Can you work these out from the model? Positions are in its coordinate system, mm. Face numbers are marked on the shaded views. A direction names the side the tool comes from. Coordinates: 2 decimals unless noted, no trailing zeros. Loops run counter-clockwise (first coordinate to the right, second up) from the corner with the lowest first, then second, coordinate; pieces in that order, holes last. Notation, with made-up numbers: (-21, 15.25) -> (-12, 15.25) arc R33 cw to (-12, 44.25) -> close; hole circle Ø11 at (55, -2.5). An arc over 180 degrees is marked (long way). Use one line per item in the form item = value. Start each with the question number.
(1) Imagine slicing it at D-D (x = 46). List the corners of the cut face in (y, z) for me.
(2) Imagine slicing it at A-A (x = 27). List the corners of the cut face in (y, z) for me, plus the area to 3 significant figures.
(3) On a 3-axis mill with a long thin cutter (end or side, diameter ignored), from which of +Z, -Z, +X, -X, +Y, -Y can I reach the whole of each face in a straight line? I mean the marked faces 1 and 2. Say none if no direction works.
(4) Imagine slicing it at B-B (y = 4.5). List the corners of the cut face in (x, z) for me, plus the area to 3 significant figures.
(5) I'm going to push flat-ended pins straight in: pin 1 (1.1 mm diameter, centred on x = 0.5, y = 13.5, fed in from +Z); pin 2 (0.6 mm diameter, centred on x = 2, y = 5, fed in from +Z); pin 3 (1.1 mm diameter, centred on x = 31, y = 27.5, fed in from +Z). Where does each tip first touch, or does it pass through?
(6) I need wall thicknesses on line 1 (X direction, y = 15.5, z = 3.5); line 2 (X direction, y = 3.5, z = 22); line 3 (Y direction, x = 6, z = 21). Which ranges of each line are inside material? Lowest first, please. Write a range as [from, to].
(7) Imagine slicing it at C-C (z = 4.75). List the corners of the cut face in (x, y) for me, plus the area to 3 significant figures.
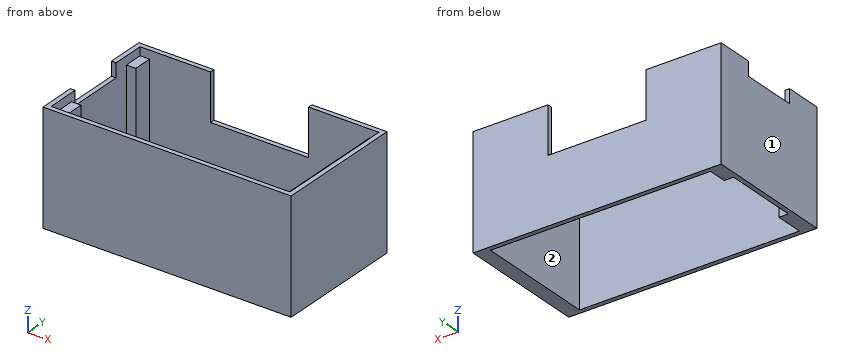
```python
from build123d import *

# Parameters (mm, degrees)
BOX006_W     = 1
BOX006_H     = 12
BOX006_DEPTH = 3
BOX005_W     = 21
BOX005_H     = 1
BOX005_DEPTH = 10
BOX004_W     = 2
BOX004_H     = 26
BOX004_DEPTH = 22.2
BOX002_W     = 2
BOX002_H     = 4
BOX002_DEPTH = 22.2
BOX001_W     = 51
BOX001_H     = 26
BOX001_DEPTH = 24
BOX_W        = 53
BOX_H        = 28
BOX_DEPTH    = 24
BOX003_W     = 2
BOX003_H     = 6
BOX003_DEPTH = 22.2


with BuildPart() as connectorcutout:
    # Box006 → Box006 (new body)
    with BuildSketch(Plane(origin=(0, 8, 21), x_dir=(1, 0, 0), z_dir=(0, 0, 1))):
        with Locations((0.5, 6)):
            Rectangle(BOX006_W, BOX006_H)
    extrude(amount=BOX006_DEPTH)


with BuildPart() as cube:
    # Box005 → Box005 (new body)
    with BuildSketch(Plane(origin=(16, 27, 14), x_dir=(1, 0, 0), z_dir=(0, 0, 1))):
        with Locations((10.5, 0.5)):
            Rectangle(BOX005_W, BOX005_H)
    extrude(amount=BOX005_DEPTH)


with BuildPart() as rightsupport:
    # Box004 → Box004 (new body)
    with BuildSketch(Plane(origin=(50, 1, 0), x_dir=(1, 0, 0), z_dir=(0, 0, 1))):
        with Locations((1, 13)):
            Rectangle(BOX004_W, BOX004_H)
    extrude(amount=BOX004_DEPTH)


with BuildPart() as topleftsupport:
    # Box002 → Box002 (new body)
    with BuildSketch(Plane(origin=(1, 23, 0), x_dir=(1, 0, 0), z_dir=(0, 0, 1))):
        with Locations((1, 2)):
            Rectangle(BOX002_W, BOX002_H)
    extrude(amount=BOX002_DEPTH)


with BuildPart() as inside:
    # Box001 → Box001 (new body)
    with BuildSketch(Plane(origin=(1, 1, 0), x_dir=(1, 0, 0), z_dir=(0, 0, 1))):
        with Locations((25.5, 13)):
            Rectangle(BOX001_W, BOX001_H)
    extrude(amount=BOX001_DEPTH)


with BuildPart() as fusion:
    # Box → Box (new body)
    with BuildSketch(Plane.XY):
        with Locations((26.5, 14)):
            Rectangle(BOX_W, BOX_H)
    extrude(amount=BOX_DEPTH)

    # Cut: cut Inside
    add(inside.part, mode=Mode.SUBTRACT)

    # Fusion: union topleftsupport
    add(topleftsupport.part)


with BuildPart() as cut002:
    # Box003 → Box003 (new body)
    with BuildSketch(Plane(origin=(1, 1, 0), x_dir=(1, 0, 0), z_dir=(0, 0, 1))):
        with Locations((1, 3)):
            Rectangle(BOX003_W, BOX003_H)
    extrude(amount=BOX003_DEPTH)

    # Fusion001: union Fusion
    add(fusion.part)

    # Fusion002: union rightsupport
    add(rightsupport.part)

    # Cut001: cut Cube
    add(cube.part, mode=Mode.SUBTRACT)

    # Cut002: cut ConnectorCutout
    add(connectorcutout.part, mode=Mode.SUBTRACT)


solid = cut002.part
```
Worked out:
q1.outline = (0, 0) -> (1, 0) -> (1, 24) -> (0, 24) -> close; (27, 0) -> (28, 0) -> (28, 24) -> (27, 24) -> close
q2.outline = (0, 0) -> (1, 0) -> (1, 24) -> (0, 24) -> close; (27, 0) -> (28, 0) -> (28, 14) -> (27, 14) -> close
q2.area = 38.0 mm2
q3.face_1 = +Z, -Z, -X, +Y, -Y
q3.face_2 = +Z, -Z
q4.outline = (0, 0) -> (3, 0) -> (3, 22.2) -> (1, 22.2) -> (1, 24) -> (0, 24) -> close; (50, 0) -> (53, 0) -> (53, 24) -> (52, 24) -> (52, 22.2) -> (50, 22.2) -> close
q4.area = 137 mm2
q5.pin_1 = 21
q5.pin_2 = 22.2
q5.pin_3 = 14
q6.line_1 = [0, 1], [50, 53]
q6.line_2 = [0, 3], [50, 53]
q6.line_3 = [0, 1], [27, 28]
q7.outline = (0, 0) -> (53, 0) -> (53, 28) -> (0, 28) -> close; hole (1, 7) -> (3, 7) -> (3, 1) -> (50, 1) -> (50, 27) -> (3, 27) -> (3, 23) -> (1, 23) -> close
q7.area = 230 mm2
